Build history of the part. All positions in model axes, mm. Face numbers are marked on the shaded views. Round coordinates to 2 decimals unless told otherwise and drop trailing zeros. Write each loop counter-clockwise with the first axis right and the second up, starting at its lowest first coordinate (ties: lowest second). Pieces come first, ordered by that corner, then holes. Notation, with made-up numbers: (65.25, 68.5) -> (74.25, 68.5) arc R9 cw to (74.25, 75.5) -> close; hole circle Ø2 at (24, -0.75). An arc over 180 degrees is marked (long way). Answer in a Markdown table with one row per item.
```python
from build123d import *

# Parameters (mm, degrees)
F0_R     = 64.7966982458
F1_DEPTH = 76.2
F2_DEPTH = 25.4
F3_D     = 101.6
F3_DEPTH = 127
F3_TIP   = 30.5237194466


with BuildPart() as f1:
    # F0 (on Right) → F1 (new body)
    with BuildSketch(Plane.YZ):
        with Locations((-8.1026245671, -10.8826834557)):
            Circle(F0_R)
    extrude(amount=F1_DEPTH)

    # F0 (on Right) → F2 (join)
    with BuildSketch(Plane.YZ):
        with Locations((-8.1026245671, -10.8826834557)):
            Circle(F0_R)
    extrude(amount=F2_DEPTH)

    # F3
    with Locations(Plane(origin=(0, 0, 0), x_dir=(0, 1, 0), z_dir=(-1, 0, 0))):
        with Locations((-8.1026245671, 10.8826834557)):
            Hole(F3_D / 2, depth=F3_DEPTH)
            with Locations((0, 0, -(F3_DEPTH + F3_TIP / 2))):  # 118° drill point
                Cone(0, F3_D / 2, F3_TIP, mode=Mode.SUBTRACT)


solid = f1.part
```
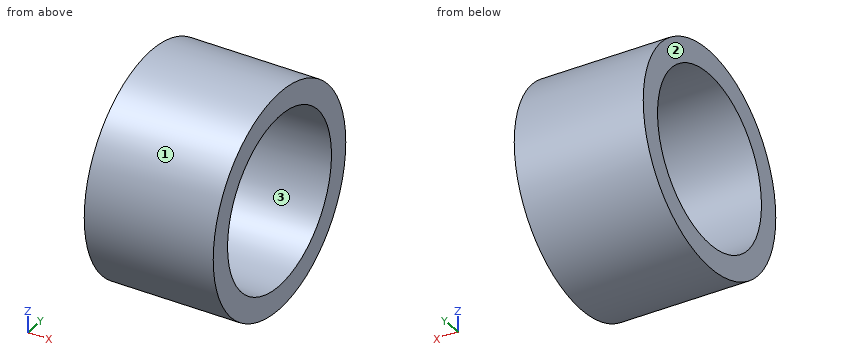
Q1. Saw through at C-C on x = 68. Write the cut outline in (y, z), plus the area to 3 significant figures.
A:
| item | result |
|---|---|
| outline | circle Ø129.59 at (-8.1, -10.88); hole circle Ø101.6 at (-8.1, -10.88) |
| area | 5,080 mm² |
Q2. Saw through at D-D on y = -64.5. Write the cut outline in (x, z).
A:
| item | result |
|---|---|
| outline | (0, -42.79) -> (76.2, -42.79) -> (76.2, 21.02) -> (0, 21.02) -> close |
Q3. Two-plate mould, pull along Y, no slides. Class the marked faces 1, 2 and 3: released by +Y, released by -Y, zero draft, split by the parting line, or undercut.
A:
| item | result |
|---|---|
| face 1 | split by the parting line |
| face 2 | zero draft |
| face 3 | undercut |
Q4. Saw through at A-A on y = -28. Write the cut outline in (x, z).
A:
| item | result |
|---|---|
| outline | (0, -72.55) -> (76.2, -72.55) -> (76.2, -57.62) -> (0, -57.62) -> close; (0, 35.86) -> (76.2, 35.86) -> (76.2, 50.78) -> (0, 50.78) -> close |
Q5. Saw through at B-B on z = -8.5. Write the cut outline in (x, y), plus the area to 3 significant figures.
A:
| item | result |
|---|---|
| outline | (0, -72.86) -> (76.2, -72.86) -> (76.2, -58.85) -> (0, -58.85) -> close; (0, 42.64) -> (76.2, 42.64) -> (76.2, 56.65) -> (0, 56.65) -> close |
| area | 2,130 mm² |
Q6. Drop flat-ended pins along their axis: P1, Ø5, axis at x = 24.5, y = -43.5, coming from the +Z side; P2, Ø1, axis at x = 62.5, y = -48, coming from the -Z side; P3, Ø8, axis at x = 18, z = 11, coming from the -Y side. Give the stop position or say it passes through.
A:
| item | result |
|---|---|
| P1 | z = 44.94 |
| P2 | z = -62.33 |
| P3 | y = -70.38 |
Q7. Wall check: line 1 (Z direction, x = 40, y = -6.5); line 2 (Z direction, x = 58.5, y = 20.5); line 3 (Y direction, x = 11, z = 4). Give the ranges that are in metal, low to high. Write a range as [from, to].
A:
| item | result |
|---|---|
| line 1 | [-75.66, -61.66], [39.89, 53.89] |
| line 2 | [-69.02, -52.87], [31.1, 47.26] |
| line 3 | [-71.17, -56.67], [40.47, 54.96] |
